CAD build for the part. Positions are in the model's coordinates, mm. A direction names the side the tool comes from. Coordinates: 2 decimals unless noted, no trailing zeros. Loops run counter-clockwise (first coordinate to the right, second up) from the corner with the lowest first, then second, coordinate; pieces in that order, holes last.
1) Which spindle directions (+Z, -Z, +X, -X, +Y, -Y) get a long thin tool onto all of the face, cutting with end or side? Do faces 4 (the flat face through (37, -82.8, 2)), 5 (the flat face through (-1, -174, 2)). Say none if no direction does.
2) Wall check: line 1 along X through (y, z) = (-127.5, 1.95); line 2 along X through (y, z) = (-67, 2.85). Give the ranges that are in metal, low to high.
3) Saw through at A-A, the plane y = -107. Write the cut outline in (x, z).
4) Saw through at B-B, the plane x = 37.5. Write the cut outline in (y, z).
5) Two-plate mould, pull along X, no slides. Class faces 1 (the flat face through (-43.5, -103, 2)), 2 (the flat face through (-1, -101, 4)), 3 (the flat face through (39.7, -87, 2)): +X half, -X half, draft (parallel to the pull), parting line (faces both ways), or undercut.
```python
from build123d import *

# Parameters (mm, degrees)
SKETCH_1_R      = 1.5
SKETCH_1_W      = 4.4
SKETCH_1_H      = 8.4
EXTRUDE_1_DEPTH = 4
SKETCH_2_W      = 87
SKETCH_2_H      = 20
EXTRUDE_2_DEPTH = 4


with BuildPart() as part:
    # 草图1 → 凸台-拉伸1 (new body)
    with BuildSketch(Plane.XY):
        Polygon((43.5, -50), (43.5, -150), (43.5, -154), (-43.5, -154), (-43.5, -150), (-43.5, -50), (-43.5, -30), (43.5, -30), align=None)
        with Locations((37.5, -147)):
            Circle(SKETCH_1_R, mode=Mode.SUBTRACT)
        with Locations((37.5, -67)):
            Circle(SKETCH_1_R, mode=Mode.SUBTRACT)
        with Locations((37.5, -107)):
            Circle(SKETCH_1_R, mode=Mode.SUBTRACT)
        with Locations((37.5, -127)):
            Rectangle(SKETCH_1_W, SKETCH_1_H, mode=Mode.SUBTRACT)
        with Locations((37.5, -87)):
            Rectangle(SKETCH_1_W, SKETCH_1_H, mode=Mode.SUBTRACT)
        with Locations((37.5, -47)):
            Rectangle(SKETCH_1_W, SKETCH_1_H, mode=Mode.SUBTRACT)
    extrude(amount=EXTRUDE_1_DEPTH)

    # 草图2 → 凸台-拉伸2 (add)
    with BuildSketch(Plane.XY.offset(4)):
        with Locations((0, -164)):
            Rectangle(SKETCH_2_W, SKETCH_2_H)
    extrude(amount=-EXTRUDE_2_DEPTH)


solid = part.part
```
Data:
1. face 4: +Z, -Z
1. face 5: +Z, -Z, +X, -X, -Y
2. line 1: x = -43.5 to 35.3, 39.7 to 43.5
2. line 2: x = -43.5 to 36, 39 to 43.5
3. outline: (-43.5, 0) - (36, 0) - (36, 4) - (-43.5, 4) - close; (39, 0) - (43.5, 0) - (43.5, 4) - (39, 4) - close
4. outline: (-174, 0) - (-148.5, 0) - (-148.5, 4) - (-174, 4) - close; (-145.5, 0) - (-131.2, 0) - (-131.2, 4) - (-145.5, 4) - close; (-122.8, 0) - (-108.5, 0) - (-108.5, 4) - (-122.8, 4) - close; (-105.5, 0) - (-91.2, 0) - (-91.2, 4) - (-105.5, 4) - close; (-82.8, 0) - (-68.5, 0) - (-68.5, 4) - (-82.8, 4) - close; (-65.5, 0) - (-51.2, 0) - (-51.2, 4) - (-65.5, 4) - close; (-42.8, 0) - (-30, 0) - (-30, 4) - (-42.8, 4) - close
5. face 1: -X half
5. face 2: draft
5. face 3: undercut
